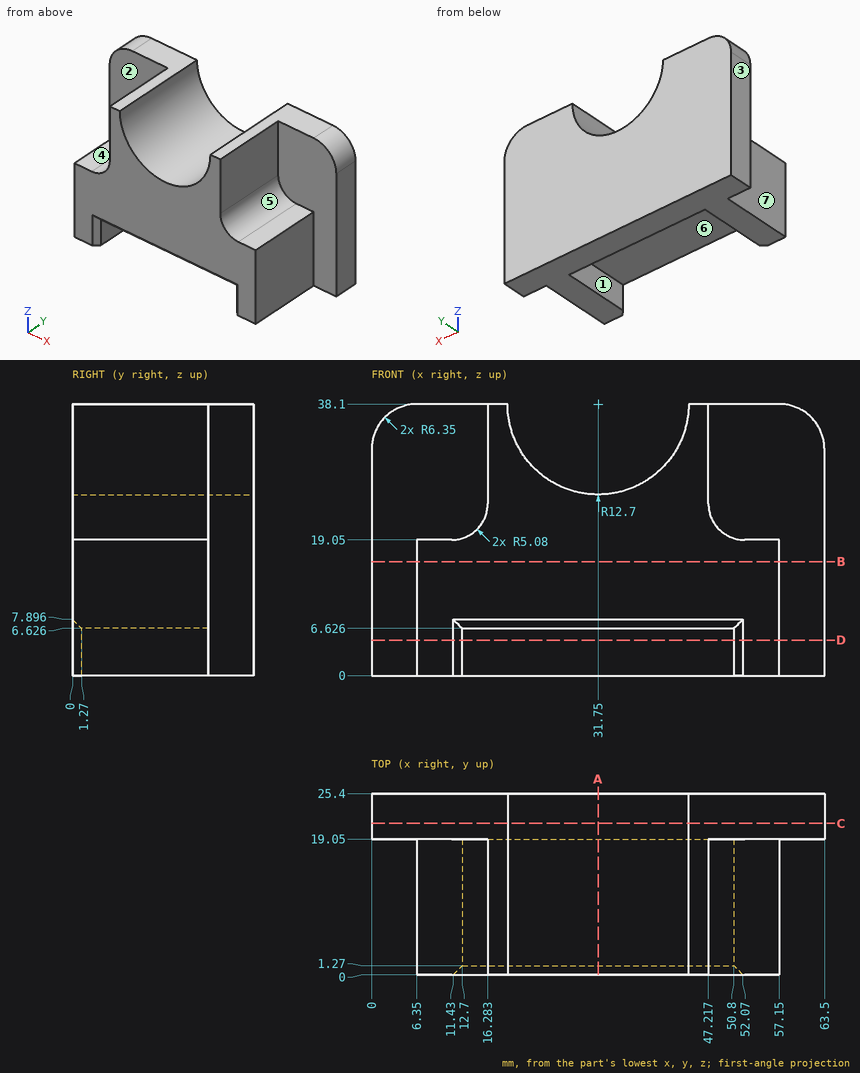
Here's the drawing with two shaded views (mm, measured from the low corner). I have some questions. A direction names the side the tool comes from. Round coordinates to 2 decimals unless told otherwise and drop trailing zeros. Write each loop counter-clockwise with the first axis right and the second up, starting at its lowest first coordinate (ties: lowest second). Pieces come first, ordered by that corner, then holes.
(1) For pin 1 (7 mm diameter, centred on y = 11, z = 34.5, fed in from +X); pin 2 (2 mm diameter, centred on x = 42.5, y = 17, fed in from -Z); pin 3 (8 mm diameter, centred on x = 11, z = 33, fed in from -Y), each with a flat end and sliding along its axis, tell me the tip position at first contact or that it passes through.
Findings below:
pin 1: stops at x = 47.22
pin 2: stops at z = 6.63
pin 3: stops at y = 19.05
(2) Suppose I cut it at C-C on y = 21.25. Write out the boundary of the cut face in (x, z).
Findings below:
outline: (0, 0) - (63.5, 0) - (63.5, 31.75) arc R6.35 ccw to (57.15, 38.1) - (44.45, 38.1) arc R12.7 cw to (19.05, 38.1) - (6.35, 38.1) arc R6.35 ccw to (0, 31.75) - close
(3) Which directions (+Z, -Z, +X, -X, +Y, -Y) give clear straight access to the entire face, cutting with the end or side of a thin tool? Please do the marked faces 4, 5, 6 and 7.
Findings below:
face 4: +Z, -X, -Y
face 5: +Z, +X, -Y
face 6: -Z, -Y
face 7: +Z, -Z, -X, -Y
(4) Thinking about a two-plate mould opening in X: for the marked faces 1, 2 and 3, which applies, +X half, -X half, draft (parallel to the pull), parting line (faces both ways), or undercut?
Findings below:
face 1: undercut
face 2: draft
face 3: -X half
(5) Suppose I cut it at D-D on z = 5. Write out the boundary of the cut face in (x, y).
Findings below:
outline: (0, 19.05) - (6.35, 19.05) - (6.35, 0) - (11.43, 0) - (12.7, 1.27) - (12.7, 19.05) - (50.8, 19.05) - (50.8, 1.27) - (52.07, 0) - (57.15, 0) - (57.15, 19.05) - (63.5, 19.05) - (63.5, 25.4) - (0, 25.4) - close
(6) If I drill on probe 1 along X at (y, z) = (9.5, 17.5); probe 2 along Z at (x, y) = (46, 12); probe 3 along Z at (x, y) = (7, 12.5), over which ranges is the centre line in solid material (lowest first)?
Findings below:
probe 1: x = 6.35 to 57.15
probe 2: z = 6.63 to 38.1
probe 3: z = 0 to 19.05
(7) Suppose I cut it at B-B on z = 16. Write out the boundary of the cut face in (x, y), and give its area (3 significant figures).
Findings below:
outline: (0, 19.05) - (6.35, 19.05) - (6.35, 0) - (57.15, 0) - (57.15, 19.05) - (63.5, 19.05) - (63.5, 25.4) - (0, 25.4) - close
area: 1,370 mm2
(8) Suppose I cut it at A-A on x = 31.75. Write out the boundary of the cut face in (y, z).
Findings below:
outline: (0, 7.9) - (1.27, 6.63) - (19.05, 6.63) - (19.05, 0) - (25.4, 0) - (25.4, 25.4) - (0, 25.4) - close
